```python
from build123d import *

# Parameters (mm, degrees)
SKETCH1_R           = 2.54
SKETCH1_R_2         = 14.2875
BOSS_EXTRUDE1_DEPTH = 3.175


with BuildPart() as part:
    # Sketch1 → Boss-Extrude1 (new body)
    with BuildSketch(Plane.XY):
        with BuildLine():
            Line((0, 0), (0, 50.8))
            Line((0, 50.8), (76.2, 50.8))
            ThreePointArc((76.2, 50.8), (101.6, 25.4), (76.2, 0))
            Line((76.2, 0), (0, 0))
        make_face()
        with Locations((12.7, 38.1)):
            Circle(SKETCH1_R, mode=Mode.SUBTRACT)
        with Locations((25.4, 38.1)):
            Circle(SKETCH1_R, mode=Mode.SUBTRACT)
        with Locations((38.1, 38.1)):
            Circle(SKETCH1_R, mode=Mode.SUBTRACT)
        with Locations((25.4, 25.4)):
            Circle(SKETCH1_R, mode=Mode.SUBTRACT)
        with Locations((38.1, 25.4)):
            Circle(SKETCH1_R, mode=Mode.SUBTRACT)
        with Locations((25.4, 12.7)):
            Circle(SKETCH1_R, mode=Mode.SUBTRACT)
        with Locations((38.1, 12.7)):
            Circle(SKETCH1_R, mode=Mode.SUBTRACT)
        with Locations((12.7, 25.4)):
            Circle(SKETCH1_R, mode=Mode.SUBTRACT)
        with Locations((12.7, 12.7)):
            Circle(SKETCH1_R, mode=Mode.SUBTRACT)
        with Locations((76.2, 25.4)):
            Circle(SKETCH1_R_2, mode=Mode.SUBTRACT)
    extrude(amount=BOSS_EXTRUDE1_DEPTH)


solid = part.part
```
Geometry check sheet. Reference: the model listing, model coordinates, mm. Round coordinates to 2 decimals unless told otherwise and drop trailing zeros. Order: outer loops, then holes, each group sorted by start corner. A loop starts at its lowest first (then second) coordinate and runs counter-clockwise, first axis right, second up. Notation, with made-up numbers: M -2.5,26 L 46.5,26 A26 ccw 46.5,44 Z; hole C 39.25,28.5 d9. An arc over 180 degrees is marked long. Answer as CSV lines item,"result".
1) Sectioned sample at D-D on y = 18.5. Record the cut outline in (x, z) (3 decimals).
Entries:
outline,"M 0,0 L 63.689,0 L 63.689,3.175 L 0,3.175 Z; M 88.711,0 L 100.645,0 L 100.645,3.175 L 88.711,3.175 Z"
2) Sectioned sample at A-A on y = 25.4. Record the cut outline in (x, z) (1 decimal), and give its area (3 significant figures).
Entries:
outline,"M 0,0 L 10.2,0 L 10.2,3.2 L 0,3.2 Z; M 15.2,0 L 22.9,0 L 22.9,3.2 L 15.2,3.2 Z; M 27.9,0 L 35.6,0 L 35.6,3.2 L 27.9,3.2 Z; M 40.6,0 L 61.9,0 L 61.9,3.2 L 40.6,3.2 Z; M 90.5,0 L 101.6,0 L 101.6,3.2 L 90.5,3.2 Z"
area,"183 mm2"
3) Mould release check, pull along Y, two halves, no side actions. Record for faces 1 (the face through (52, 26, 3.175)), 2 (the face through (39, 0, 2)), 3 (the face through (26.77, 27.54, 1.57)): +Y half, -Y half, draft (parallel to the pull), parting line (faces both ways), or undercut.
Entries:
face 1,"draft"
face 2,"-Y half"
face 3,"undercut"
4) Thickness scan on probe 1 along Y at (x, z) = (25.4, 2.4); probe 2 along Y at (x, z) = (36, 0.35); probe 3 along X at (y, z) = (40, 0.65). Record the ranges inside material, lowest first. Write a range as [from, to].
Entries:
probe 1,"[0, 10.16], [15.24, 22.86], [27.94, 35.56], [40.64, 50.8]"
probe 2,"[0, 11.27], [14.13, 23.97], [26.83, 36.67], [39.53, 50.8]"
probe 3,"[0, 11.01], [14.39, 23.71], [27.09, 36.41], [39.79, 96.98]"
5) Gauge pin test, flat ends, axial feed: pin 1 Ø3 at (x, y) = (25.4, 25.4) entering from -Z; pin 2 Ø8 at (x, y) = (38.1, 38.1) entering from +Z (3 decimals); pin 3 Ø1 at (x, z) = (84, 0.5) entering from +Y. Record the tip position at first contact, or that the pin passes through.
Entries:
pin 1,"through"
pin 2,"z = 3.175"
pin 3,"y = 49.73"
6) Sectioned sample at B-B on x = 25.4. Record the cut outline in (y, z) (3 decimals), and give its area (3 significant figures).
Entries:
outline,"M 0,0 L 10.16,0 L 10.16,3.175 L 0,3.175 Z; M 15.24,0 L 22.86,0 L 22.86,3.175 L 15.24,3.175 Z; M 27.94,0 L 35.56,0 L 35.56,3.175 L 27.94,3.175 Z; M 40.64,0 L 50.8,0 L 50.8,3.175 L 40.64,3.175 Z"
area,"113 mm2"
7) Sectioned sample at C-C on z = 0.85. Give the number of separate pieces and of enclosed holes in the cut face, and give its area (3 significant figures).
Entries:
separate pieces,"1"
enclosed holes,"10"
area,"4,060 mm2"
